Geometry: see drawing. Coordinates: mm, zero at the bounding-box minimum. Coordinates: 2 decimals unless noted, no trailing zeros. Order: outer loops, then holes, each group sorted by start corner. A loop starts at its lowest first (then second) coordinate and runs counter-clockwise, first axis right, second up. Notation, with made-up numbers: M 18,61.25 L 36,61.25 A15 cw 36,90.25 Z; hole C 6,16.5 d6. An arc over 180 degrees is marked long. One line per item, written item: value.
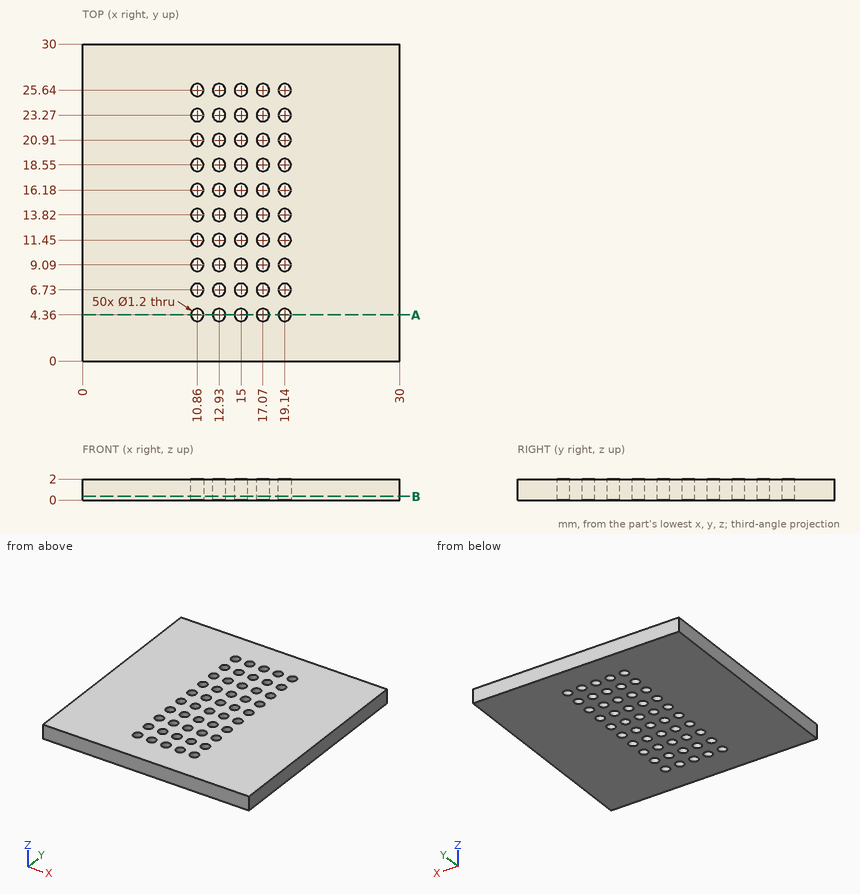
(1) Ray query, line 1 (X direction, y = 18.55, z = 1.6); line 2 (X direction, y = 4, z = 1.15). Return the intervals inside material, ascending. Write a range as from..to.
Data:
line 1: x = 0..10.26, 11.46..12.33, 13.53..14.4, 15.6..16.47, 17.67..18.54, 19.74..30
line 2: x = 0..10.38, 11.34..12.45, 13.41..14.52, 15.48..16.59, 17.55..18.66, 19.62..30
(2) Cut plane A-A on y = 4.36. Output: boundary loops of the cut face in (x, z), plus the area to 3 significant figures.
Data:
outline: M 0,0 L 10.26,0 L 10.26,2 L 0,2 Z; M 11.46,0 L 12.33,0 L 12.33,2 L 11.46,2 Z; M 13.53,0 L 14.4,0 L 14.4,2 L 13.53,2 Z; M 15.6,0 L 16.47,0 L 16.47,2 L 15.6,2 Z; M 17.67,0 L 18.54,0 L 18.54,2 L 17.67,2 Z; M 19.74,0 L 30,0 L 30,2 L 19.74,2 Z
area: 48.0 mm2
(3) Cut plane B-B on z = 0.35. Give the number of separate pieces and of enclosed holes in the cut face, plus the area to 3 significant figures.
Data:
separate pieces: 1
enclosed holes: 50
area: 843 mm2
